The listing builds one solid part. Answer for the finished solid, in the listing's coordinates (mm). A direction names the side the tool comes from. Give positions to 0.01 mm unless a question says otherwise; leave off trailing zeros. Write each loop counter-clockwise with the first axis right and the second up, starting at its lowest first coordinate (ties: lowest second). Pieces come first, ordered by that corner, then holes. Notation, with made-up numbers: (24, -30) - (72, -30) arc R24 cw to (72, 6) - close; hole circle Ø11 at (-16, 73.25). An arc over 180 degrees is marked (long way). Return JSON: item names as keys, results as strings.
from build123d import *

# Parameters (mm, degrees)
SKETCH_1_R          = 2
EXTRUDE_1_DEPTH     = 12
CHAMFER_1_SIZE      = 0.2
CUT_EXTRUDE_1_DEPTH = 5


with BuildPart() as part:
    # 草图1 → 凸台-拉伸1 (new body)
    with BuildSketch(Plane(origin=(0, 0, 0), x_dir=(1, 0, 0), z_dir=(0, 1, 0))):
        with Locations(Location((0, 0, 0), (0, 0, 270))):
            Circle(SKETCH_1_R)
    extrude(amount=EXTRUDE_1_DEPTH)

    # 倒角1
    chamfer_1_edges = [part.edges().sort_by_distance(p)[0] for p in [
        (0, 0, -2),
        (0, 12, -2),
    ]]
    chamfer(chamfer_1_edges, length=CHAMFER_1_SIZE)

    # 草图2 → 切除-拉伸1 (cut)
    with BuildSketch(Plane(origin=(0, 12, 0), x_dir=(1, 0, 0), z_dir=(0, 1, 0))):
        Polygon((-1.154700538, 0), (-0.577350269, -1), (0.577350269, -1), (1.154700538, 0), (0.577350269, 1), (-0.577350269, 1), align=None)
    extrude(amount=-CUT_EXTRUDE_1_DEPTH, mode=Mode.SUBTRACT)


solid = part.part
Item 1: A cutting plane is placed at C-C on y = 2.75. Determine the outline of the cut face in (x, z).
Answer below:
{"outline": "circle Ø4 at (0, 0)"}
Item 2: A cutting plane is placed at B-B on x = 0. Determine the outline of the cut face in (y, z), then the cut area to 3 significant figures.
Answer below:
{"outline": "(0, -1.8) - (0.2, -2) - (11.8, -2) - (12, -1.8) - (12, -1) - (7, -1) - (7, 1) - (12, 1) - (12, 1.8) - (11.8, 2) - (0.2, 2) - (0, 1.8) - close", "area": "37.9 mm²"}
Item 3: The mould has two halves that part along Z. Classify faces 1 (the face through (-1, 12, 1)), 2 (the face through (0, 10, 1)), 3 (the face through (0, 7, 0)), 4 (the face through (-2, 6, 0)): +Z half, -Z half, draft (parallel to the pull), parting line (faces both ways), or undercut.
Answer below:
{"face 1": "draft", "face 2": "undercut", "face 3": "undercut", "face 4": "parting line"}
Item 4: A flat-ended cylindrical pin translates along its axis: P1, Ø2, axis at x = 1.5, y = 5, coming from the +Z side. Find the tip coordinate at first contact, or state that the pin passes through.
Answer below:
{"P1": "stops at z = 1.94"}
Item 5: For faces 5 (the face through (0.87, 9.54, -0.49)), 6 (the face through (0, 0, 0)), determine the directions among +Z, -Z, +X, -X, +Y, -Y from which every point of the face is accessible in a straight line to the end or side of a thin tool.
Answer below:
{"face 5": "+Y", "face 6": "+Z, -Z, +X, -X, -Y"}
Item 6: A cutting plane is placed at A-A on y = 7.75. Determine the outline of the cut face in (x, z).
Answer below:
{"outline": "circle Ø4 at (0, 0); hole (-1.15, 0) - (-0.58, -1) - (0.58, -1) - (1.15, 0) - (0.58, 1) - (-0.58, 1) - close"}
Item 7: Consider L1, parallel to X at y = 10.25, z = -0.5; L2, parallel to Z at x = 0.7, y = 11; L3, parallel to Y at x = 0.45, z = 0.7. Determine where each line is inside the solid, lowest interval first.
Answer below:
{"L1": "x = -1.94 to -0.87, 0.87 to 1.94", "L2": "z = -1.87 to -0.79, 0.79 to 1.87", "L3": "y = 0 to 7"}
